Verification items for the finished model (mm, model axes). Face numbers are marked on the shaded views. A direction names the side the tool comes from. Coordinates: 2 decimals unless noted, no trailing zeros. Order: outer loops, then holes, each group sorted by start corner. A loop starts at its lowest first (then second) coordinate and runs counter-clockwise, first axis right, second up. Notation, with made-up numbers: M -11,77.5 L 37,77.5 A23 cw 37,95.5 Z; hole C 15,67.25 d7. An arc over 180 degrees is marked long. Answer as a JSON object with one key per item and string values. Group by question number.
(1) Gauge pin test, flat ends, axial feed: pin 1 Ø1.5 at (x, z) = (7.67, 3) entering from +Y; pin 2 Ø1 at (x, z) = (-10.5, 4.5) entering from +Y; pin 3 Ø1 at (y, z) = (41, 4.5) entering from -X. Record the tip position at first contact, or that the pin passes through.
(2) Cross-section at A-A (x = -10.5). Enter the section's corners in (y, z), plus the area to 3 significant figures.
(3) Cross-section at C-C (y = 43.5). Enter the section's corners in (x, z).
(4) Material ranges on line 1 (X direction, y = -14.5, z = 3); line 2 (Y direction, x = -13.5, z = 2.4); line 3 (X direction, y = 50, z = 5.35), recorded low to high.
(5) Access from +Z, -Z, +X, -X, +Y, -Y to the whole of each face (thin tool, end or side, straight path). Record for the marked faces 1 and 2.
(6) Cross-section at B-B (y = 14). Enter the section's corners in (x, z).
from build123d import *

# Parameters (mm, degrees)
SKETCH_1_R                       = 3
EXTRUDE_1_DEPTH                  = 6
SKETCH_2_W                       = 16
SKETCH_2_H                       = 26
SKETCH_2_R                       = 1.6
EXTRUDE_2_DEPTH                  = 6
FILLET_2_R                       = 10
FILLET_3_R                       = 2
SKETCH_3_W                       = 39.771534619
SKETCH_3_H                       = 15.568928143
CUT_EXTRUDE_1_DEPTH              = 16
HOLE_WIZARD_M3_1_D               = 2.5
HOLE_WIZARD_M3_1_DEPTH           = 7.5
HOLE_WIZARD_M3_1_TIP             = 0.751075774
CUT_EXTRUDE_2_DEPTH              = 7
EXTRUDE_3_DEPTH                  = 6
HOLE_WIZARD_M3_3_D               = 2.5
HOLE_WIZARD_M3_3_DEPTH           = 7.5
HOLE_WIZARD_M3_3_TIP             = 0.751075774
HOLE_WIZARD_M3_3_ON_FACE_2_D     = 2.5
HOLE_WIZARD_M3_3_ON_FACE_2_DEPTH = 7.5
HOLE_WIZARD_M3_3_ON_FACE_2_TIP   = 0.751075774


with BuildPart() as part:
    # 草图1 → 凸台-拉伸1 (new body)
    with BuildSketch(Plane.XY):
        with BuildLine():
            Line((19.167299473, 7.939450352), (-3.832700527, 47.776618926))
            Line((-3.832700527, 47.776618926), (-3.832700527, 49.489431847))
            ThreePointArc((-3.832700527, 49.489431847), (-11.832700527, 57.489431847), (-19.832700527, 49.489431847))
            Line((-19.832700527, 49.489431847), (-19.832700527, 43.489431847))
            Line((-19.832700527, 43.489431847), (3.167299473, 3.652263273))
            Line((3.167299473, 3.652263273), (3.167299473, -56.491330266))
            Line((3.167299473, -56.491330266), (19.167299473, -56.491330266))
            Line((19.167299473, -56.491330266), (19.167299473, 7.939450352))
        make_face()
        with Locations((-11.832700527, 49.489431847)):
            Circle(SKETCH_1_R, mode=Mode.SUBTRACT)
    extrude(amount=EXTRUDE_1_DEPTH)

    # 草图2 → 凸台-拉伸2 (add)
    with BuildSketch(Plane.XZ.offset(56.491330266)):
        with Locations((11.167299473, -7)):
            Rectangle(SKETCH_2_W, SKETCH_2_H)
        with Locations((7.167299473, -8)):
            Circle(SKETCH_2_R, mode=Mode.SUBTRACT)
        with Locations((15.167299473, -15)):
            Circle(SKETCH_2_R, mode=Mode.SUBTRACT)
    extrude(amount=-EXTRUDE_2_DEPTH)

    # 圆角2
    fillet_2_edges = [part.edges().sort_by_distance(p)[0] for p in [
        (-19.832700527, 43.489431847, 3),
    ]]
    fillet(fillet_2_edges, radius=FILLET_2_R)

    # 圆角3
    fillet_3_edges = [part.edges().sort_by_distance(p)[0] for p in [
        (3.167299473, -53.491330266, -20),
        (19.167299473, -53.491330266, -20),
    ]]
    fillet(fillet_3_edges, radius=FILLET_3_R)

    # 草图3 → 切除-拉伸1 (cut)
    with BuildSketch(Plane(origin=(19.167299473, 0, 0), x_dir=(0, 0, -1), z_dir=(1, 0, 0))):
        with Locations((8.066218502, -58.275794338)):
            Rectangle(SKETCH_3_W, SKETCH_3_H)
    extrude(amount=-CUT_EXTRUDE_1_DEPTH, mode=Mode.SUBTRACT)

    # M3 螺纹孔1
    with Locations(Plane(origin=(0, -50.491330266, 0), x_dir=(-1, 0, 0), z_dir=(0, -1, 0))):
        with Locations((-7.667299473, -3), (-14.667299473, -3)):
            Hole(HOLE_WIZARD_M3_1_D / 2, depth=HOLE_WIZARD_M3_1_DEPTH)
            with Locations((0, 0, -(HOLE_WIZARD_M3_1_DEPTH + HOLE_WIZARD_M3_1_TIP / 2))):  # 118° drill point
                Cone(0, HOLE_WIZARD_M3_1_D / 2, HOLE_WIZARD_M3_1_TIP, mode=Mode.SUBTRACT)

    # 草图9 → 切除-拉伸2 (cut, through all)
    with BuildSketch(Plane.XY.offset(6)):
        Polygon((10.439222522, 23.056923084), (29.925755937, 19.338586327), (19.167299473, -5.491330266), align=None)
    extrude(amount=-CUT_EXTRUDE_2_DEPTH, mode=Mode.SUBTRACT)

    # 草图12 → 凸台-拉伸3 (add)
    with BuildSketch(Plane.XY.offset(6)):
        Polygon((-4.328668805, 16.635661183), (3.167299473, -7.882546288), (3.167299473, 3.652263273), align=None)
    extrude(amount=-EXTRUDE_3_DEPTH)

    # M3 螺纹孔3
    with Locations(Plane(origin=(14.240054683, 10.624961257, 3), x_dir=(-0.292371705, 0.956304756, 0), z_dir=(0.956304756, 0.292371705, 0))):
        with Locations((0, 0)):
            Hole(HOLE_WIZARD_M3_3_D / 2, depth=HOLE_WIZARD_M3_3_DEPTH)
            with Locations((0, 0, -(HOLE_WIZARD_M3_3_DEPTH + HOLE_WIZARD_M3_3_TIP / 2))):  # 118° drill point
                Cone(0, HOLE_WIZARD_M3_3_D / 2, HOLE_WIZARD_M3_3_TIP, mode=Mode.SUBTRACT)

    # M3 螺纹孔3 on face 2
    with Locations(Plane(origin=(16.579028321, 2.974523209, 3), x_dir=(-0.292371907, 0.956304694, 0), z_dir=(0.956304694, 0.292371907, 0))):
        with Locations((0, 0)):
            Hole(HOLE_WIZARD_M3_3_ON_FACE_2_D / 2, depth=HOLE_WIZARD_M3_3_ON_FACE_2_DEPTH)
            with Locations((0, 0, -(HOLE_WIZARD_M3_3_ON_FACE_2_DEPTH + HOLE_WIZARD_M3_3_ON_FACE_2_TIP / 2))):  # 118° drill point
                Cone(0, HOLE_WIZARD_M3_3_ON_FACE_2_D / 2, HOLE_WIZARD_M3_3_ON_FACE_2_TIP, mode=Mode.SUBTRACT)


solid = part.part
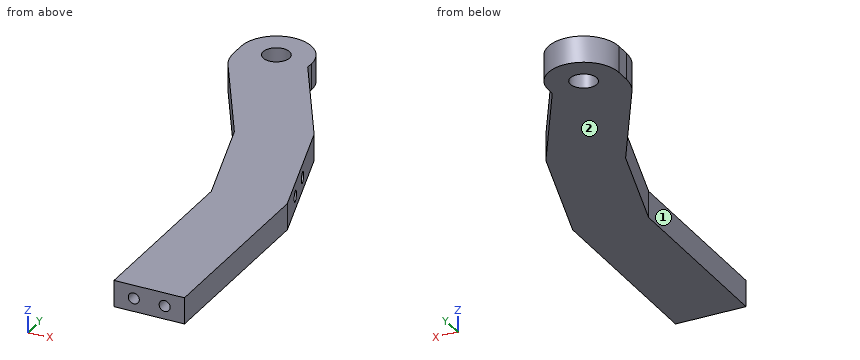
Taken from the geometry:
{
 "1": {"pin 1": "stops at y = 29.15", "pin 2": "stops at y = 57.45", "pin 3": "stops at x = -18.68"},
 "2": {"outline": "M 27.32,0 L 46.8,0 L 46.8,6 L 27.32,6 Z; M 52.18,0 L 57.38,0 L 57.38,6 L 52.18,6 Z", "area": "148 mm²"},
 "3": {"outline": "M -19.47,0 L -1.36,0 L -1.36,6 L -19.47,6 Z"},
 "4": {"line 1": "x = 3.17 to 19.17", "line 2": "y = 32.52 to 47, 51.98 to 57.31", "line 3": "x = -19.82 to -14.79, -8.88 to -3.85"},
 "5": {"face 1": "+Z, -Z, -X, -Y", "face 2": "-Z, +X, -X, +Y, -Y"},
 "6": {"outline": "M -3.52,0 L 13.21,0 L 13.21,6 L -3.52,6 Z"}
}
